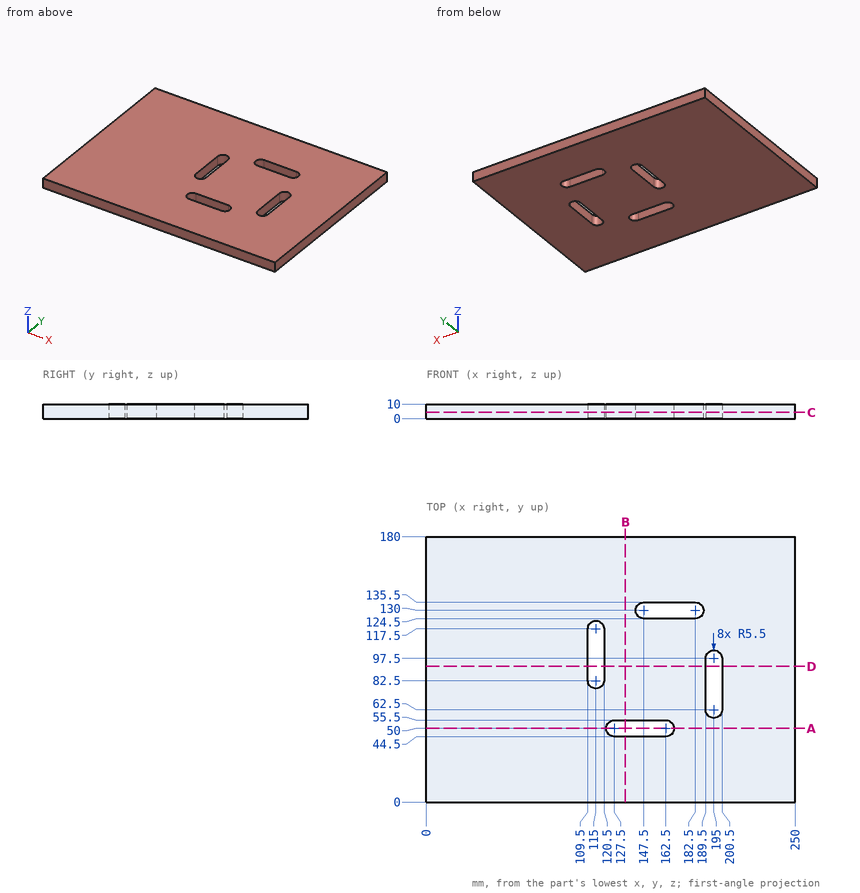
Input: dimensioned drawing with shaded views. Units: mm. Origin: part minimum x, y, z. Round coordinates to 2 decimals unless told otherwise and drop trailing zeros. Loops run counter-clockwise (first coordinate to the right, second up) from the corner with the lowest first, then second, coordinate; pieces in that order, holes last. Notation, with made-up numbers: (-13, -22) -> (2, -22) arc R7 cw to (2, -13) -> close; hole circle Ø4 at (42.25, 58.25). An arc over 180 degrees is marked (long way). Use one line per item in the form item = value. Start each with the question number.
1) Section C-C on z = 4.25. Output: boundary loops of the cut face in (x, y).
2) Section D-D on y = 92. Output: boundary loops of the cut face in (x, z), then the cut area to 3 significant figures.
3) Section A-A on y = 50. Output: boundary loops of the cut face in (x, z), then the cut area to 3 significant figures.
4) Section B-B on x = 135. Output: boundary loops of the cut face in (y, z), then the cut area to 3 significant figures.
5) Line query: L1, parallel to Y at x = 158, z = 0.75; L2, parallel to X at y = 114, z = 2.5; L3, parallel to X at y = 67, z = 5.5. Output: solid intervals per line, ascending.
Response:
q1.outline = (0, 0) -> (250, 0) -> (250, 180) -> (0, 180) -> close; hole (109.5, 82.5) arc R5.5 ccw to (120.5, 82.5) -> (120.5, 117.5) arc R5.5 ccw to (109.5, 117.5) -> close; hole (127.5, 44.5) -> (162.5, 44.5) arc R5.5 ccw to (162.5, 55.5) -> (127.5, 55.5) arc R5.5 ccw to start; hole (147.5, 124.5) -> (182.5, 124.5) arc R5.5 ccw to (182.5, 135.5) -> (147.5, 135.5) arc R5.5 ccw to start; hole (189.5, 62.5) arc R5.5 ccw to (200.5, 62.5) -> (200.5, 97.5) arc R5.5 ccw to (189.5, 97.5) -> close
q2.outline = (0, 0) -> (109.5, 0) -> (109.5, 10) -> (0, 10) -> close; (120.5, 0) -> (189.5, 0) -> (189.5, 10) -> (120.5, 10) -> close; (200.5, 0) -> (250, 0) -> (250, 10) -> (200.5, 10) -> close
q2.area = 2,280 mm^2
q3.outline = (0, 0) -> (122, 0) -> (122, 10) -> (0, 10) -> close; (168, 0) -> (250, 0) -> (250, 10) -> (168, 10) -> close
q3.area = 2,040 mm^2
q4.outline = (0, 0) -> (44.5, 0) -> (44.5, 10) -> (0, 10) -> close; (55.5, 0) -> (180, 0) -> (180, 10) -> (55.5, 10) -> close
q4.area = 1,690 mm^2
q5.L1 = 0 to 44.5, 55.5 to 124.5, 135.5 to 180
q5.L2 = 0 to 109.5, 120.5 to 250
q5.L3 = 0 to 189.5, 200.5 to 250
